Source: CAD feature listing. Evaluate the final solid. Frame: model axes, mm. Give positions to 0.01 mm unless a question says otherwise; leave off trailing zeros. Write each loop counter-clockwise with the first axis right and the second up, starting at its lowest first coordinate (ties: lowest second). Pieces come first, ordered by that corner, then holes. Notation, with made-up numbers: (34.5, 85.5) -> (54.5, 85.5) arc R14 cw to (54.5, 103.5) -> close; hole circle Ø11 at (14, 34). An arc over 180 degrees is marked (long way). Write item = value, one per line.
from build123d import *

# Parameters (mm, degrees)
SKETCH17_R              = 165.1
BOSS_EXTRUDE1_DEPTH     = 1.27
DOME2_FACE_RADIUS       = 165.1
DOME2_HEIGHT            = 20.32
CUT_EXTRUDE1_REACH      = 236.483
CUT_EXTRUDE1_END_RADIUS = 680.87875
SKETCH18_R              = 8.89


# Read off the part's stored shape, not the designer's step: Shell2
with BuildPart() as part:
    # Sketch17 → Boss-Extrude1 (new body)
    with BuildSketch(Plane.XY):
        Circle(SKETCH17_R)
    extrude(amount=BOSS_EXTRUDE1_DEPTH)

    # Dome2: a dome of height H over a round flat face of radius A is a cap of a sphere of radius (A * A + H * H) / (2 * H)
    dome2_r = (DOME2_FACE_RADIUS * DOME2_FACE_RADIUS + DOME2_HEIGHT * DOME2_HEIGHT) / (2 * DOME2_HEIGHT)
    dome2_base = Plane((0, 0, 1.27), z_dir=(0, 0, 1))
    with Locations(dome2_base.offset(DOME2_HEIGHT - dome2_r)):
        dome2_ball = Sphere(dome2_r, mode=Mode.PRIVATE)
    add(split(dome2_ball, bisect_by=dome2_base, keep=Keep.TOP, mode=Mode.PRIVATE))

    # Shell2 outline → Shell2 (revolve, cut)
    with BuildSketch(Plane.XZ):
        with BuildLine():
            Line((0, 0), (159.630210195, -1e-07))
            ThreePointArc((159.630210195, -1e-07), (80.381444548, 14.27066321), (0, 19.05))
            Line((0, 19.05), (0, 0))
        make_face()
    revolve(axis=Axis((0, 0, 0), (0, 0, 1)), mode=Mode.SUBTRACT)

    # Cut-Extrude1: up to this sphere (the profile starts inside it)
    cut_extrude1_end = Location((0, 0, -659.28875)) * Sphere(CUT_EXTRUDE1_END_RADIUS, mode=Mode.PRIVATE)
    # Sketch18 → Cut-Extrude1 (cut, up to the surface)
    with BuildSketch(Plane.XY, mode=Mode.PRIVATE) as cut_extrude1_sk1:
        Circle(SKETCH18_R)
    cut_extrude1_tool1 = extrude(cut_extrude1_sk1.sketch, amount=CUT_EXTRUDE1_REACH, mode=Mode.PRIVATE) & cut_extrude1_end
    add(cut_extrude1_tool1.solids().sort_by_distance((0, 0, 0))[0], mode=Mode.SUBTRACT)


solid = part.part
1) Material intervals for L1, parallel to Z at x = -30, y = -14.5; L2, parallel to Z at x = -24, y = -14, sorted ascending.
Computed:
L1 = 18.23 to 20.77
L2 = 18.48 to 21.02
2) Cut plane C-C (y = -83). Return the cut outline in (x, z).
Computed:
outline = (-142.72, 0) -> (-136.36, 0) arc R673.24 cw to (136.36, 0) -> (142.72, 0) -> (142.72, 1.27) arc R675.8 ccw to (-142.72, 1.27) -> close
3) Cut plane A-A (x = 0). Return the cut outline in (y, z), then the cut area to 3 significant figures.
Computed:
outline = (-165.1, 0) -> (-159.63, 0) arc R678.34 cw to (-8.89, 18.99) -> (-8.89, 21.53) arc R680.88 ccw to (-165.1, 1.27) -> close; (8.89, 18.99) arc R678.34 cw to (159.63, 0) -> (165.1, 0) -> (165.1, 1.27) arc R680.88 ccw to (8.89, 21.53) -> close
area = 795 mm²
4) Contact query for a flat-ended pin moving along its axis: pin 1 (12 mm diameter, centred on y = -126.5, z = 19, fed in from +X). Output: stop coordinate, or through.
Computed:
pin_1 = through
5) Draft query along X for faces 1 (the cylindrical face through (-35.79, -161.174, 0.626)), 2 (the flat face through (-86, 135, 0)), 3 (the cylindrical face through (-1.93, -8.68, 20.24)). Return one class per face: pulls with the +X half, pulls with the -X half, needs draft (parallel to the pull), parting line crosses it, or undercut.
Computed:
face_1 = parting line crosses it
face_2 = needs draft
face_3 = undercut
6) Cut plane D-D (x = 51.5). Return the cut outline in (y, z).
Computed:
outline = (-156.86, 0) -> (-151.09, 0) arc R676.38 cw to (151.09, 0) -> (156.86, 0) -> (156.86, 1.27) arc R678.93 ccw to (-156.86, 1.27) -> close
